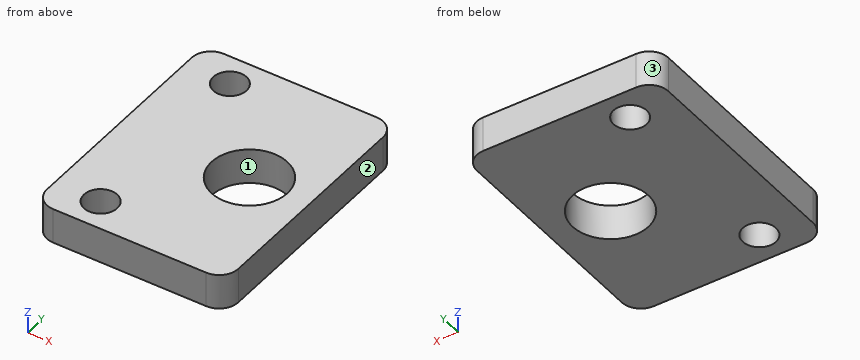
Autodesk Inventor part; units mm, degrees
ref_plane "YZ Plane" through (0, 0, 0) normal (1, 0, 0) x (0, 1, 0)
ref_plane "XZ Plane" through (0, 0, 0) normal (0, 1, 0) x (-1, 0, 0)
ref_plane "XY Plane" through (0, 0, 0) normal (0, 0, 1) x (1, 0, 0)
sketch "Sketch1" plane through (0, 0, 0) normal (0, 0, 1) x (1, 0, 0)
  line L0 (0, 29.337) -> (0, -29.337)
  line L1 (-22.225, 0) -> (22.225, 0)
  line L2 (15.875, -20.955) -> (-15.875, -20.955)
  line L3 (-15.875, -20.955) -> (-15.875, 20.955)
  line L4 (-15.875, 20.955) -> (15.875, 20.955)
  line L5 (15.875, 20.955) -> (15.875, -20.955)
  line L6 (15.875, -20.955) -> (-15.875, 20.955) construction
  line L7 (-15.875, -20.955) -> (15.875, 20.955) construction
  point P0 (0, 0)
  point P1 (-8.255, 15.875)
  point P2 (-8.255, -15.875)
  point P3 (5.715, 0)
  dimension "d0" = 41.91
  dimension "d1" = 31.75
  dimension "d2" = 31.75
  dimension "d3" = 15.875
  dimension "d4" = 7.62
  dimension "d5" = 10.16
extrude "Extrusion1" add sketch "Sketch1" against normal blind 5.842
hole "Hole1" at (-8.255, 15.875, 0) at (-8.255, -15.875, 0) direction (0, 0, -1) diameter 5.5118 end through all
hole "Hole2" at (5.715, 0, 0) direction (0, 0, -1) diameter 12.573 end through all
fillet "Fillet1" radius 3.175 4 edges at (-15.875, -20.955, -2.921) (15.875, -20.955, -2.921) (15.875, 20.955, -2.921) (-15.875, 20.955, -2.921)
Part model, mm, in its own coordinate system. Face numbers are marked on the shaded views. Coordinates: 2 decimals unless noted, no trailing zeros. Loops run counter-clockwise (first coordinate to the right, second up) from the corner with the lowest first, then second, coordinate; pieces in that order, holes last. Notation, with made-up numbers: (37.5, 14.5) - (73.5, 14.5) arc R14 cw to (73.5, 19.5) - close; hole circle Ø6 at (49, 46.25). An arc over 180 degrees is marked (long way). Write item = value, one per line. Start each with the question number.
Item 1: Flat gauge pin, fed straight in: pin 1 Ø16.5 at (x, y) = (5.715, 0) entering from +Z. Where does the tip first touch, or does it go through?
Item 2: Wall check: L1, parallel to Y at x = -10.5, z = -4.3 (3 decimals); L2, parallel to X at y = 0, z = -1.6 (1 decimal); L3, parallel to X at y = 1.5, z = -3.4 (3 decimals). Give the ranges that are in metal, low to high. Write a range as from..to.
Item 3: Mould opens along Y. For the marked faces 1, 2 and 3 say: released by +Y, released by -Y, zero draft, split by the parting line, or undercut.
Item 4: Cut at A-A, the plane x = 3. Give the cut face in (y, z) (3 decimals).
Item 5: Cut at C-C, the plane z = -4.95. State how many separate pieces and enclosed holes the cut face has, and give its area (3 significant figures).
Item 6: Cut at B-B, the plane y = -17. Give the cut face in (x, z) (3 decimals).
The answers:
q1.pin_1 = 0
q2.L1 = -20.955..-17.473, -14.277..14.277, 17.473..20.955
q2.L2 = -15.9..-0.6, 12..15.9
q2.L3 = -15.875..-0.39, 11.82..15.875
q3.face_1 = undercut
q3.face_2 = zero draft
q3.face_3 = released by +Y
q4.outline = (-20.955, -5.842) - (-5.67, -5.842) - (-5.67, 0) - (-20.955, 0) - close; (5.67, -5.842) - (20.955, -5.842) - (20.955, 0) - (5.67, 0) - close
q5.separate_pieces = 1
q5.enclosed_holes = 3
q5.area = 1,150 mm2
q6.outline = (-15.875, -5.842) - (-10.771, -5.842) - (-10.771, 0) - (-15.875, 0) - close; (-5.739, -5.842) - (15.875, -5.842) - (15.875, 0) - (-5.739, 0) - close
